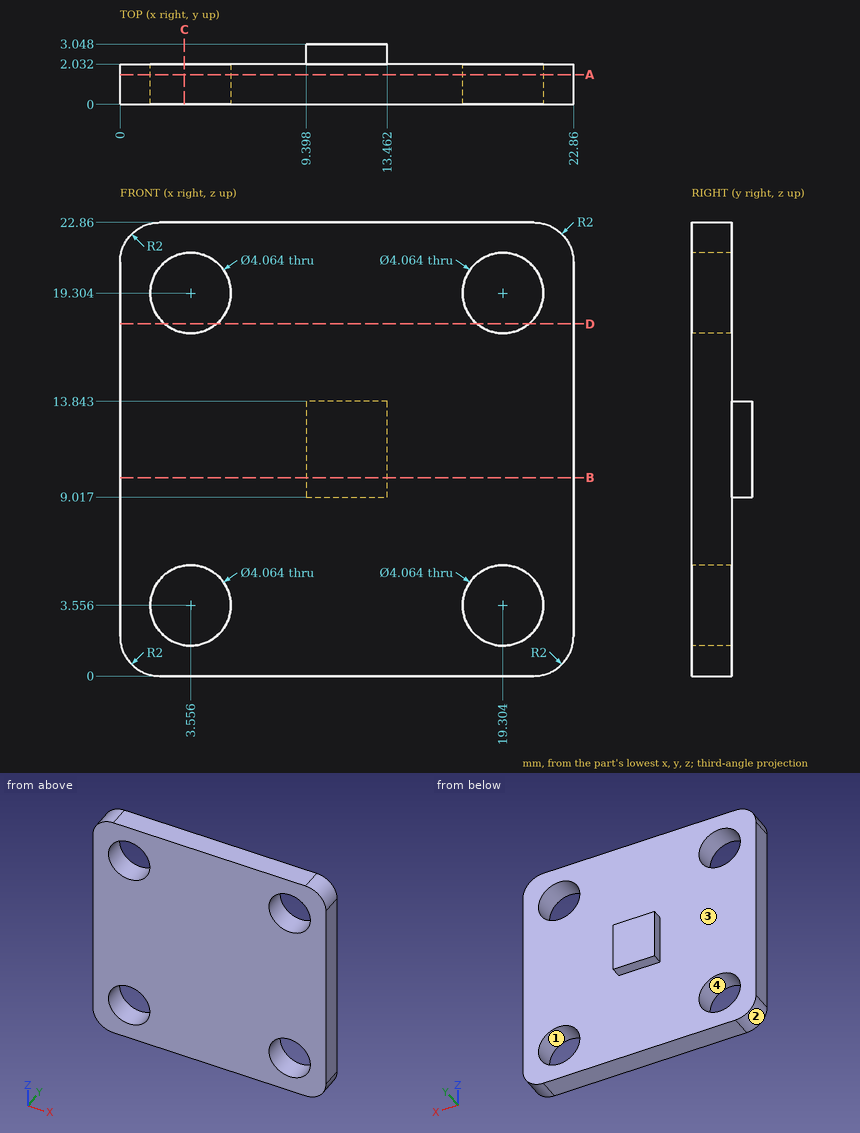
Geometry check sheet. Reference: drawing and pictorial views, mm from the part's lowest x, y, z. Round coordinates to 2 decimals unless told otherwise and drop trailing zeros. Order: outer loops, then holes, each group sorted by start corner. A loop starts at its lowest first (then second) coordinate and runs counter-clockwise, first axis right, second up.
Q1. Draft check along X on the marked faces 1, 2, 3 and 4. Enter one of: pulls with the +X half, pulls with the -X half, needs draft (parallel to the pull), parting line crosses it, or undercut.
Filled sheet:
face 1: undercut
face 2: pulls with the -X half
face 3: needs draft
face 4: undercut
Q2. Cross-section at C-C, the plane x = 3.25. Enter the section's corners in (y, z), plus the area to 3 significant figures.
Filled sheet:
outline: (0, 0) - (2.03, 0) - (2.03, 1.55) - (0, 1.55) - close; (0, 5.56) - (2.03, 5.56) - (2.03, 17.3) - (0, 17.3) - close; (0, 21.31) - (2.03, 21.31) - (2.03, 22.86) - (0, 22.86) - close
area: 30.1 mm2
Q3. Cross-section at B-B, the plane z = 10. Enter the section's corners in (x, y), plus the area to 3 significant figures.
Filled sheet:
outline: (0, 0) - (22.86, 0) - (22.86, 2.03) - (13.46, 2.03) - (13.46, 3.05) - (9.4, 3.05) - (9.4, 2.03) - (0, 2.03) - close
area: 50.6 mm2
Q4. Cross-section at D-D, the plane z = 17.75. Enter the section's corners in (x, y), plus the area to 3 significant figures.
Filled sheet:
outline: (0, 0) - (2.25, 0) - (2.25, 2.03) - (0, 2.03) - close; (4.87, 0) - (17.99, 0) - (17.99, 2.03) - (4.87, 2.03) - close; (20.61, 0) - (22.86, 0) - (22.86, 2.03) - (20.61, 2.03) - close
area: 35.8 mm2
Q5. Cross-section at A-A, the plane y = 1.5. Enter the section's corners in (x, z).
Filled sheet:
outline: (0, 2) arc R2 ccw to (2, 0) - (20.86, 0) arc R2 ccw to (22.86, 2) - (22.86, 20.86) arc R2 ccw to (20.86, 22.86) - (2, 22.86) arc R2 ccw to (0, 20.86) - close; hole circle Ø4.06 at (3.56, 3.56); hole circle Ø4.06 at (3.56, 19.3); hole circle Ø4.06 at (19.3, 3.56); hole circle Ø4.06 at (19.3, 19.3)
Q6. Depth check by flat-ended pin: P1, Ø0.5, axis at y = 2.5, z = 11.5, coming from the -X side; P2, Ø1, axis at x = 4.5, z = 4, coming from the -Y side; P3, Ø3, axis at x = 7.5, z = 5, coming from the +Y side; P4, Ø0.5, axis at x = 11, y = 2.5, coming from the -Z side. Enter the tip coordinate at first touch or a pass-through.
Filled sheet:
P1: stops at x = 9.4
P2: passes through
P3: stops at y = 2.03
P4: stops at z = 9.02
Q7. Scan lines: L1, parallel to Z at x = 19.75, y = 2; L2, parallel to Z at x = 4.5, y = 0.95; L3, parallel to Y at x = 1.5, z = 17. Record each from-to range of solid material in increasing order.
Filled sheet:
L1: z = 0 to 1.57, 5.54 to 17.32, 21.29 to 22.86
L2: z = 0 to 1.76, 5.36 to 17.5, 21.1 to 22.86
L3: y = 0 to 2.03
